from build123d import *

# Parameters (mm, degrees)
F0_R            = 4.05
F1_DEPTH        = 10
F2_R            = 5
F4_D            = 3.7973
F4_CSINK_D      = 7.7978
F4_CSINK_ANGLE  = 82
F5_W            = 1
F5_H            = 12
F6_DEPTH        = 0.4
F8_DEPTH        = 25
F10_D           = 3
F10_CBORE_D     = 6.5
F10_CBORE_DEPTH = 3


with BuildPart() as f1:
    # F0 (on Top) → F1 (new body)
    with BuildSketch(Plane.XY):
        Polygon((67.5994434953, -8.2149432153), (-62.4005565047, -8.2149432153), (-62.4005565047, -32.2149432153), (-28.9914757013, -32.2149432153), (-28.9914757013, -20.2149432153), (34.1903626919, -20.2149432153), (34.1903626919, -32.2149432153), (67.5994434953, -32.2149432153), align=None)
        with Locations((-47.4005565047, -20.2149432153)):
            Circle(F0_R, mode=Mode.SUBTRACT)
        with Locations((52.5994434953, -20.2149432153)):
            Circle(F0_R, mode=Mode.SUBTRACT)
    extrude(amount=F1_DEPTH)

    # F2
    f2_edges = [f1.edges().sort_by_distance(p)[0] for p in [
        (34.190363, -32.214943, 5),
        (-28.991476, -32.214943, 5),
    ]]
    fillet(f2_edges, radius=F2_R)

    # F4 (through all)
    with Locations(Plane.XZ.offset(20.2149432153)):
        with Locations((-18.9914757013, 5), (24.1903626919, 5)):
            CounterSinkHole(F4_D / 2, F4_CSINK_D / 2, counter_sink_angle=F4_CSINK_ANGLE)

    # F5 (on face) → F6 (join)
    with BuildSketch(Plane.XY.offset(10)):
        with Locations((2.5994434953, -14.2149432153)):
            Rectangle(F5_W, F5_H)
    extrude(amount=F6_DEPTH)

    # F7 (on face) → F8 (cut)
    with BuildSketch(Plane.XY.offset(10)):
        with BuildLine():
            ThreePointArc((56.6417200816, -19.9649432153), (56.6475121814, -20.0898835784), (56.6494434953, -20.2149432153))
            ThreePointArc((56.6494434953, -20.2149432153), (56.6475121814, -20.3400028521), (56.6417200816, -20.4649432153))
            Line((56.6417200816, -20.4649432153), (67.5994434953, -20.4649432153))
            Line((67.5994434953, -20.4649432153), (67.5994434953, -19.9649432153))
            Line((67.5994434953, -19.9649432153), (56.6417200816, -19.9649432153))
        make_face()
        with BuildLine():
            Line((-51.442833091, -19.9649432153), (-62.4005565047, -19.9649432153))
            Line((-62.4005565047, -19.9649432153), (-62.4005565047, -20.4649432153))
            Line((-62.4005565047, -20.4649432153), (-51.442833091, -20.4649432153))
            ThreePointArc((-51.442833091, -20.4649432153), (-51.4505565047, -20.2149432153), (-51.442833091, -19.9649432153))
        make_face()
        with BuildLine():
            Line((-51.442833091, -20.4649432153), (-51.442833091, -19.9649432153))
            ThreePointArc((-51.442833091, -19.9649432153), (-51.4505565047, -20.2149432153), (-51.442833091, -20.4649432153))
        make_face()
        with BuildLine():
            ThreePointArc((56.6417200816, -20.4649432153), (56.6475121814, -20.3400028521), (56.6494434953, -20.2149432153))
            ThreePointArc((56.6494434953, -20.2149432153), (56.6475121814, -20.0898835784), (56.6417200816, -19.9649432153))
            Line((56.6417200816, -19.9649432153), (56.6417200816, -20.4649432153))
        make_face()
    extrude(amount=-F8_DEPTH, mode=Mode.SUBTRACT)

    # F10 (through all)
    with Locations(Plane.XZ.offset(32.2149432153)):
        with Locations((61.5994434953, 5), (-56.4005565047, 5)):
            CounterBoreHole(F10_D / 2, F10_CBORE_D / 2, F10_CBORE_DEPTH)


solid = f1.part
Could you check a few things on this model? Use its own coordinates, in mm. A direction names the side the tool comes from. Give positions to 0.01 mm unless a question says otherwise; leave off trailing zeros. Order: outer loops, then holes, each group sorted by start corner. A loop starts at its lowest first (then second) coordinate and runs counter-clockwise, first axis right, second up.
1. Suppose I cut it at B-B (x = -47). List the corners of the cut face in (y, z) for me.
2. We'd pull the mould along Y, two halves only. Please class faces 1 (the flat face through (67.599, -26, 5)), 2 (the flat face through (2, -20.215, 5)), 3 (the flat face through (63.3, -20.465, 5.1)): pulls with the +Y half, pulls with the -Y half, needs draft (parallel to the pull), parting line crosses it, or undercut.
3. I need wall thicknesses on L1, parallel to X at y = -10.5, z = 5.25; L2, parallel to X at y = -11.25, z = 6.25; L3, parallel to X at y = -26.75, z = 9. Which ranges of each line are inside material? Lowest first, please.
4. For faces 4 (the flat face through (4, -8.215, 5)), 5 (the flat face through (-31, -17, 10)), 6 (the flat face through (53, -32.215, 5)), 7 (the cylindrical face through (58.353, -30.736, 5.143)), 8 (the flat face through (-58.2, -20.465, 5.1)), which set-ups out of +Z, -Z, +X, -X, +Y, -Y let a thin tool reach every point of the face, with its end or its side?
5. Will these pins go through, and if not, where does the flat tip stop? P1, Ø7, axis at x = -33, y = -19, coming from the +Z side; P2, Ø2.5, axis at x = -56.4, z = 5, coming from the +Y side; P3, Ø5, axis at x = 61.6, z = 5, coming from the -Y side; P4, Ø3, axis at x = -7, z = 8, coming from the -Y side.
6. Suppose I cut it at D-D (x = 8). List the corners of the cut face in (y, z) for me.
7. Suppose I cut it at C-C (z = 5). Give the number of separate pieces and of enclosed holes in the cut face, plus the area to 3 significant figures.
8. Suppose I cut it at A-A (y = -12). List the corners of the cut face in (x, z) for me, plus the area to 3 significant figures.
Solved:
1. outline: (-32.21, 0) - (-24.25, 0) - (-24.25, 10) - (-32.21, 10) - close; (-16.18, 0) - (-8.21, 0) - (-8.21, 10) - (-16.18, 10) - close
2. face 1: needs draft
2. face 2: pulls with the -Y half
2. face 3: undercut
3. L1: x = -62.4 to -57.88, -54.92 to -20.87, -17.11 to 22.31, 26.07 to 60.12, 63.08 to 67.6
3. L2: x = -62.4 to -57.23, -55.57 to -20.42, -17.56 to 22.76, 25.62 to 60.77, 62.43 to 67.6
3. L3: x = -62.4 to -28.99, 34.19 to 67.6
4. face 4: +Z, -Z, +X, -X, +Y
4. face 5: +Z, -X, +Y, -Y
4. face 6: +Z, -Z, +X, -X, -Y
4. face 7: -Y
4. face 8: +Z, -Z, -X
5. P1: stops at z = 10
5. P2: passes through
5. P3: stops at y = -29.21
5. P4: stops at y = -20.21
6. outline: (-20.21, 0) - (-8.21, 0) - (-8.21, 10) - (-20.21, 10) - close
7. separate pieces: 7
7. enclosed holes: 0
7. area: 1,970 mm2
8. outline: (-62.4, 0) - (67.6, 0) - (67.6, 10) - (3.1, 10) - (3.1, 10.4) - (2.1, 10.4) - (2.1, 10) - (-62.4, 10) - close; hole circle Ø3 at (-56.4, 5); hole circle Ø3.8 at (-18.99, 5); hole circle Ø3.8 at (24.19, 5); hole circle Ø3 at (61.6, 5)
8. area: 1,260 mm2
